Read the model definition and answer for the solid it produces. Units are mm, in the model's axes. A direction names the side the tool comes from. Round coordinates to 2 decimals unless told otherwise and drop trailing zeros. Loops run counter-clockwise (first coordinate to the right, second up) from the corner with the lowest first, then second, coordinate; pieces in that order, holes last. Notation, with made-up numbers: (51, 87) - (70, 87) arc R6 ccw to (70, 98) - close; hole circle Ø4 at (58.5, -7.75). An arc over 180 degrees is marked (long way). Use CSV: the item, a comma, the result in double quotes. Start each with the question number.
1. Determine the mould class of faces 1 (the flat face through (0, 22, -5.25)), 2 (the flat face through (24, 22, 1)), 3 (the cylindrical face through (-30.296, 17.581, 0.986)) for opening direction X: +X half, -X half, draft (parallel to the pull), parting line (faces both ways), or undercut.
2. Consider line 1 along Y through (x, z) = (25.45, 0.85); line 2 along X through (y, z) = (16, -6.75); line 3 along X through (y, z) = (12, -3.75). Determine where each line is inside the solid, lowest interval first.
3. Find section C-C (y = 29.5). Give the vertices of the cut face in (x, z).
4. A tool of negligible diameter and unlimited length cuts with its end or side. For faces 4 (the flat face through (-23, 18, 0)), 5 (the flat face through (-24, 22, 1)), 6 (the flat face through (12.5, 22, -7)), from which of +Z, -Z, +X, -X, +Y, -Y can it reach the whole face along a straight path? Write none if from no direction.
5. Find section D-D (x = 9). Give the vertices of the cut face in (y, z), and give its area (3 significant figures).
6. Find section A-A (y = 17.5). Give the vertices of the cut face in (x, z).
7. Given pin 1 Ø1 at (x, z) = (-24, 1) entering from +Y; pin 2 Ø2.5 at (x, y) = (-24, 18) entering from -Z; pin 3 Ø3 at (y, z) = (17.5, -4) entering from +X, each flat-ended and moving along its own axis, determine where each tip first touches the part or whether it passes through.
8. Find section B-B (x = 25.45). Give the vertices of the cut face in (y, z), and give its area (3 significant figures).
from build123d import *

# Parameters (mm, degrees)
EXTRUDE001_DEPTH                     = 44
EXTRUDE001_ONTO_SKETCH001_ROLL_ANGLE = 90
SKETCH_R                             = 1.85
EXTRUDE_DEPTH                        = 2


with BuildPart() as extrude001:
    # Sketch001 as drawn → Extrude001 (new)
    with BuildSketch(Plane.XY):
        Polygon((-20.25, 0), (20.25, 0), (20.25, -8), (12.5, -8), (12.5, -5.25), (-12.5, -5.25), (-12.5, -8), (-20.25, -8), align=None)
    extrude(amount=-EXTRUDE001_DEPTH)


with BuildPart() as extrude001_1:
    # Extrude001 onto Sketch001 roll: moved
    add(extrude001.part.rotate(Axis((0, 0, 0), (1, 0, 0)), EXTRUDE001_ONTO_SKETCH001_ROLL_ANGLE))


with BuildPart() as extrude001_2:
    # Extrude001 onto Sketch001 placement: moved
    add(extrude001_1.part)


with BuildPart() as fusion:
    # Sketch → Extrude (new body)
    with BuildSketch(Plane.XY):
        with BuildLine():
            Line((-20.25, 44), (-20.25, 22))
            Line((-20.25, 22), (-27.25, 22))
            ThreePointArc((-27.25, 22), (-30.296648, 17.5), (-27.25, 13))
            Line((-27.25, 13), (-20.25, 13))
            Line((-20.25, 13), (-20.25, 0))
            Line((-20.25, 0), (20.25, 0))
            Line((20.25, 0), (20.25, 13))
            Line((20.25, 13), (27.25, 13))
            ThreePointArc((27.25, 13), (30.296648, 17.5), (27.25, 22))
            Line((27.25, 22), (20.25, 22))
            Line((20.25, 22), (20.25, 44))
            Line((20.25, 44), (-20.25, 44))
        make_face()
        with Locations((-25.45, 17.5)):
            Circle(SKETCH_R, mode=Mode.SUBTRACT)
        with Locations((25.45, 17.5)):
            Circle(SKETCH_R, mode=Mode.SUBTRACT)
    extrude(amount=EXTRUDE_DEPTH)

    # Fusion: union Extrude001
    add(extrude001_2.part)


solid = fusion.part
Filled sheet:
1,face 1,"undercut"
1,face 2,"draft"
1,face 3,"-X half"
2,line 1,"y = 13 to 15.65, 19.35 to 22"
2,line 2,"x = -20.25 to -12.5, 12.5 to 20.25"
2,line 3,"x = -20.25 to 20.25"
3,outline,"(-20.25, -8) - (-12.5, -8) - (-12.5, -5.25) - (12.5, -5.25) - (12.5, -8) - (20.25, -8) - (20.25, 2) - (-20.25, 2) - close"
4,face 4,"-Z, -X, +Y, -Y"
4,face 5,"+Z, -Z, -X, +Y"
4,face 6,"-Z, +Y, -Y"
5,outline,"(0, -5.25) - (44, -5.25) - (44, 2) - (0, 2) - close"
5,area,"319 mm²"
6,outline,"(-30.3, 0) - (-27.3, 0) - (-27.3, 2) - (-30.3, 2) - close; (-23.6, 0) - (-20.25, 0) - (-20.25, -8) - (-12.5, -8) - (-12.5, -5.25) - (12.5, -5.25) - (12.5, -8) - (20.25, -8) - (20.25, 0) - (23.6, 0) - (23.6, 2) - (-23.6, 2) - close; (27.3, 0) - (30.3, 0) - (30.3, 2) - (27.3, 2) - close"
7,pin 1,"stops at y = 22"
7,pin 2,"stops at z = 0"
7,pin 3,"stops at x = 20.25"
8,outline,"(13, 0) - (15.65, 0) - (15.65, 2) - (13, 2) - close; (19.35, 0) - (22, 0) - (22, 2) - (19.35, 2) - close"
8,area,"10.6 mm²"
